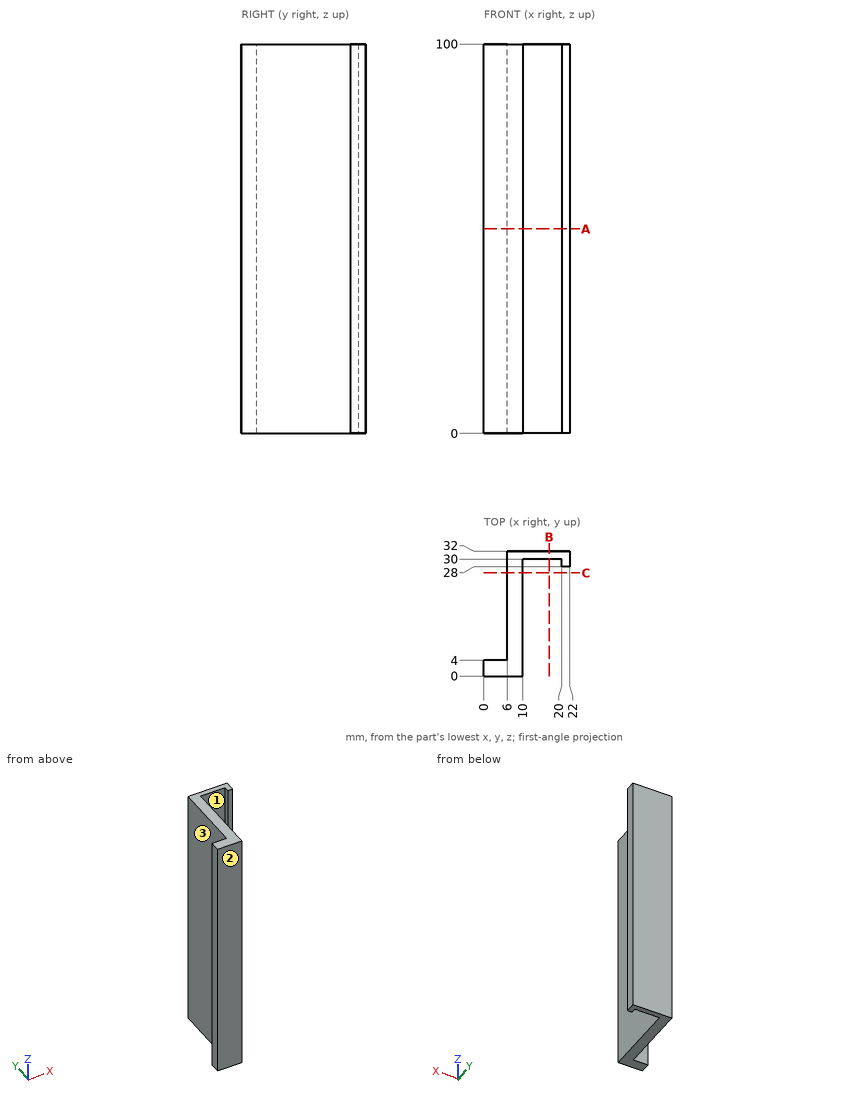
Design review of the part shown in the three views and the two pictorial views. Dimensions are in mm from the part's minimum x, y and z. Round coordinates to 2 decimals unless told otherwise and drop trailing zeros. Order: outer loops, then holes, each group sorted by start corner. A loop starts at its lowest first (then second) coordinate and runs counter-clockwise, first axis right, second up. Notation, with made-up numbers: (-9.5, 42.5) -> (-1.5, 42.5) arc R26 cw to (-1.5, 74.5) -> close; hole circle Ø5 at (7.25, -19.75). An arc over 180 degrees is marked (long way). Write item = value, one per line. Start each with the question number.
1) To check wall thickness, follow line 1 (X direction, y = 29, z = 17); line 2 (X direction, y = 16.5, z = 52); line 3 (Y direction, x = 20.5, z = 84). State the ranges of each line that lie inside material, in increasing order. Write a range as from..to.
2) Take a section at B-B on x = 16.75. State the section outline as (y, z) points, plus the area to 3 significant figures.
3) Insertion check: pin 1 (1 mm diameter, centred on x = 21, z = 59.5, fed in from -Y); pin 2 (2 mm diameter, centred on y = 14, z = 73.5, fed in from +X); pin 3 (5 mm diameter, centred on x = 14, z = 33, fed in from -Y). Each pin has a flat end and moves straight along its axis. Give the tip position at first contact, or say it passes through.
4) The part is to be moulded in two halves that separate along X. For the marked faces 1, 2 and 3, say which applies: +X half, -X half, draft (parallel to the pull), parting line (faces both ways), or undercut.
5) Take a section at A-A on z = 52.5. State the section outline as (x, y) points, plus the area to 3 significant figures.
6) Take a section at C-C on y = 26.5. State the section outline as (x, z) points, plus the area to 3 significant figures.
Verdict:
q1.line_1 = 6..10, 20..22
q1.line_2 = 6..10
q1.line_3 = 28..32
q2.outline = (30, 0) -> (32, 0) -> (32, 100) -> (30, 100) -> close
q2.area = 200 mm2
q3.pin_1 = 28
q3.pin_2 = 10
q3.pin_3 = 30
q4.face_1 = undercut
q4.face_2 = draft
q4.face_3 = -X half
q5.outline = (0, 0) -> (10, 0) -> (10, 30) -> (20, 30) -> (20, 28) -> (22, 28) -> (22, 32) -> (6, 32) -> (6, 4) -> (0, 4) -> close
q5.area = 180 mm2
q6.outline = (6, 0) -> (10, 0) -> (10, 100) -> (6, 100) -> close
q6.area = 400 mm2
